Part model, mm, in its own coordinate system. Face numbers are marked on the shaded views. A direction names the side the tool comes from. Round coordinates to 2 decimals unless told otherwise and drop trailing zeros. Write each loop counter-clockwise with the first axis right and the second up, starting at its lowest first coordinate (ties: lowest second). Pieces come first, ordered by that corner, then holes.
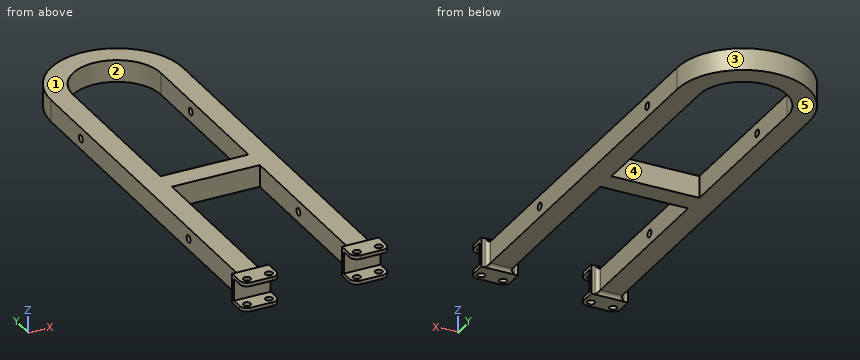
```python
from build123d import *

# Parameters (mm, degrees)
SKETCH1_R               = 5
BOSS_EXTRUDE1_DEPTH     = 50
SKETCH2_W               = 30
SKETCH2_H               = 30
CUT_EXTRUDE1_DEPTH      = 639.479639456
SKETCH3_W               = 30
SKETCH3_H               = 30
SKETCH3_W_2             = 5
SKETCH3_H_2             = 35
CUT_EXTRUDE2_DEPTH      = 642.526499842
FILLET1_R               = 5
SKETCH4_R               = 5
CUT_EXTRUDE3_DEPTH      = 639.10755363
SKETCH5_W               = 30
SKETCH5_H               = 30
BOSS_EXTRUDE2_DEPTH     = 120
SKETCH6_W               = 41.881061045
SKETCH6_H               = 38.598384764
CUT_EXTRUDE4_DEPTH      = 642.156182221
SKETCH7_W               = 50
SKETCH7_H               = 40
BOSS_EXTRUDE3_DEPTH     = 30
SKETCH8_R               = 5
CUT_EXTRUDE5_DEPTH      = 617.973459721
FILLET2_R               = 10
SKETCH9_W               = 30
SKETCH9_H               = 25
CUT_EXTRUDE6_DEPTH      = 642.156182221
CUT_EXTRUDE7_DEPTH      = 639.10755363
CUT_EXTRUDE7_DEPTH_BACK = 639.10755363
SKETCH10_R              = 5


with BuildPart() as part:
    # Sketch1 → Boss-Extrude1 (new body)
    with BuildSketch(Plane.XY):
        with BuildLine():
            Line((90, 17.5), (90, 517.5))
            ThreePointArc((90, 517.5), (0, 607.5), (-90, 517.5))
            Line((-90, 517.5), (-90, 17.5))
            Line((-90, 17.5), (-100, 17.5))
            Line((-100, 17.5), (-100, -7.5))
            ThreePointArc((-100, -7.5), (-97.071067812, -14.571067812), (-90, -17.5))
            Line((-90, -17.5), (-60, -17.5))
            ThreePointArc((-60, -17.5), (-52.928932188, -14.571067812), (-50, -7.5))
            Line((-50, -7.5), (-50, 17.5))
            Line((-50, 17.5), (-60, 17.5))
            Line((-60, 17.5), (-60, 517.5))
            ThreePointArc((-60, 517.5), (0, 577.5), (60, 517.5))
            Line((60, 517.5), (60, 17.5))
            Line((60, 17.5), (50, 17.5))
            Line((50, 17.5), (50, -7.5))
            ThreePointArc((50, -7.5), (52.928932188, -14.571067812), (60, -17.5))
            Line((60, -17.5), (90, -17.5))
            ThreePointArc((90, -17.5), (97.071067812, -14.571067812), (100, -7.5))
            Line((100, -7.5), (100, 17.5))
            Line((100, 17.5), (90, 17.5))
        make_face()
        with Locations((90, -7.5)):
            Circle(SKETCH1_R, mode=Mode.SUBTRACT)
        with Locations((60, -7.5)):
            Circle(SKETCH1_R, mode=Mode.SUBTRACT)
        with Locations((-90, -7.5)):
            Circle(SKETCH1_R, mode=Mode.SUBTRACT)
        with Locations((-60, -7.5)):
            Circle(SKETCH1_R, mode=Mode.SUBTRACT)
    extrude(amount=BOSS_EXTRUDE1_DEPTH)

    # Sketch2 → Cut-Extrude1 (cut, through all)
    with BuildSketch(Plane(origin=(90, 0, 0), x_dir=(0, 0, -1), z_dir=(1, 0, 0))):
        with BuildLine():
            Line((-50, 17.5), (-45, 17.5))
            ThreePointArc((-45, 17.5), (-41.464466094, 18.964466094), (-40, 22.5))
            Line((-40, 22.5), (-40, 607.5))
            Line((-40, 607.5), (-50, 607.5))
            Line((-50, 607.5), (-50, 17.5))
        make_face()
        with Locations((-25, -2.5)):
            Rectangle(SKETCH2_W, SKETCH2_H)
        with BuildLine():
            Line((-5, 17.5), (0, 17.5))
            Line((0, 17.5), (0, 607.5))
            Line((0, 607.5), (-10, 607.5))
            Line((-10, 607.5), (-10, 22.5))
            ThreePointArc((-10, 22.5), (-8.535533906, 18.964466094), (-5, 17.5))
        make_face()
    extrude(amount=-CUT_EXTRUDE1_DEPTH, mode=Mode.SUBTRACT)

    # Sketch3 → Cut-Extrude2 (cut, through all)
    with BuildSketch(Plane(origin=(100, 0, 0), x_dir=(0, 0, -1), z_dir=(1, 0, 0))):
        with Locations((-25, -2.5)):
            Rectangle(SKETCH3_W, SKETCH3_H)
        with Locations((-47.5, 0)):
            Rectangle(SKETCH3_W_2, SKETCH3_H_2)
        with Locations((-2.5, 0)):
            Rectangle(SKETCH3_W_2, SKETCH3_H_2)
    extrude(amount=-CUT_EXTRUDE2_DEPTH, mode=Mode.SUBTRACT)

    # Fillet1
    # the kernel refuses this fillet: 5 mm, written as the material it adds along each edge
    with BuildSketch(Plane(origin=(-90, 17.5, 5), x_dir=(-1, 0, 0), z_dir=(0, 0, 1))) as fillet1_piece_1_section:
        with BuildLine():
            CenterArc((FILLET1_R, -FILLET1_R), FILLET1_R, 90, 90)
            Line((0, -FILLET1_R), (0, 0))
            Line((0, 0), (FILLET1_R, 0))
        make_face()
    fillet1_piece_1 = extrude(amount=40, mode=Mode.PRIVATE)
    fillet1_piece_1 = fillet1_piece_1 - Plane(origin=(-91.427889151, 22.5, 45), x_dir=(0, -1, 0), z_dir=(1, 0, 0)) * Cylinder(5, 101, mode=Mode.PRIVATE)
    fillet1_piece_1 = fillet1_piece_1 - Plane(origin=(-91.427889151, 22.5, 5), x_dir=(0, 0, 1), z_dir=(1, 0, 0)) * Cylinder(5, 101, mode=Mode.PRIVATE)
    add(fillet1_piece_1)
    with BuildSketch(Plane(origin=(60, 17.5, 5), x_dir=(-1, 0, 0), z_dir=(0, 0, 1))) as fillet1_piece_2_section:
        with BuildLine():
            CenterArc((FILLET1_R, -FILLET1_R), FILLET1_R, 90, 90)
            Line((0, -FILLET1_R), (0, 0))
            Line((0, 0), (FILLET1_R, 0))
        make_face()
    fillet1_piece_2 = extrude(amount=40, mode=Mode.PRIVATE)
    fillet1_piece_2 = fillet1_piece_2 - Plane(origin=(58.572110849, 22.5, 5), x_dir=(0, 0, 1), z_dir=(1, 0, 0)) * Cylinder(5, 101, mode=Mode.PRIVATE)
    fillet1_piece_2 = fillet1_piece_2 - Plane(origin=(58.572110849, 22.5, 45), x_dir=(0, -1, 0), z_dir=(1, 0, 0)) * Cylinder(5, 101, mode=Mode.PRIVATE)
    add(fillet1_piece_2)
    with BuildSketch(Plane(origin=(-60, 17.5, 5), x_dir=(1, 0, 0), z_dir=(0, 0, 1))) as fillet1_piece_3_section:
        with BuildLine():
            CenterArc((FILLET1_R, FILLET1_R), FILLET1_R, 180, 90)
            Line((0, FILLET1_R), (0, 0))
            Line((0, 0), (FILLET1_R, 0))
        make_face()
    fillet1_piece_3 = extrude(amount=40, mode=Mode.PRIVATE)
    fillet1_piece_3 = fillet1_piece_3 - Plane(origin=(-58.572110849, 22.5, 45), x_dir=(0, -1, 0), z_dir=(1, 0, 0)) * Cylinder(5, 101, mode=Mode.PRIVATE)
    fillet1_piece_3 = fillet1_piece_3 - Plane(origin=(-58.572110849, 22.5, 5), x_dir=(0, 0, 1), z_dir=(1, 0, 0)) * Cylinder(5, 101, mode=Mode.PRIVATE)
    add(fillet1_piece_3)
    with BuildSketch(Plane(origin=(90, 17.5, 5), x_dir=(0, 1, 0), z_dir=(0, 0, 1))) as fillet1_piece_4_section:
        with BuildLine():
            CenterArc((FILLET1_R, -FILLET1_R), FILLET1_R, 90, 90)
            Line((0, -FILLET1_R), (0, 0))
            Line((0, 0), (FILLET1_R, 0))
        make_face()
    fillet1_piece_4 = extrude(amount=40, mode=Mode.PRIVATE)
    fillet1_piece_4 = fillet1_piece_4 - Plane(origin=(91.427889151, 22.5, 5), x_dir=(0, 0, 1), z_dir=(1, 0, 0)) * Cylinder(5, 101, mode=Mode.PRIVATE)
    fillet1_piece_4 = fillet1_piece_4 - Plane(origin=(91.427889151, 22.5, 45), x_dir=(0, -1, 0), z_dir=(1, 0, 0)) * Cylinder(5, 101, mode=Mode.PRIVATE)
    add(fillet1_piece_4)

    # Sketch4 → Cut-Extrude3 (cut, through all)
    with BuildSketch(Plane(origin=(90, 0, 0), x_dir=(0, 0, -1), z_dir=(1, 0, 0))):
        with Locations(Location((-25, 152.5, 0), (0, 0, 90))):
            Circle(SKETCH4_R)
    extrude(amount=-CUT_EXTRUDE3_DEPTH, mode=Mode.SUBTRACT)

    # Sketch5 → Boss-Extrude2 (add)
    with BuildSketch(Plane(origin=(-60, 0, 0), x_dir=(0, 0, -1), z_dir=(1, 0, 0))):
        with Locations((-25, 270)):
            Rectangle(SKETCH5_W, SKETCH5_H)
    extrude(amount=BOSS_EXTRUDE2_DEPTH)

    # Sketch6 → Cut-Extrude4 (cut, through all)
    with BuildSketch(Plane(origin=(100, 0, 0), x_dir=(0, 0, -1), z_dir=(1, 0, 0))):
        with Locations((-24.059469477, -1.799192382)):
            Rectangle(SKETCH6_W, SKETCH6_H)
    extrude(amount=-CUT_EXTRUDE4_DEPTH, mode=Mode.SUBTRACT)

    # Sketch7 → Boss-Extrude3 (add)
    with BuildSketch(Plane.XZ.offset(-17.5)):
        with Locations((-75, 25)):
            Rectangle(SKETCH7_W, SKETCH7_H)
        with Locations((75, 25)):
            Rectangle(SKETCH7_W, SKETCH7_H)
    extrude(amount=BOSS_EXTRUDE3_DEPTH)

    # Sketch8 → Cut-Extrude5 (cut, through all)
    with BuildSketch(Plane.XY.offset(45)):
        with Locations((-90, -2.5)):
            Circle(SKETCH8_R)
        with Locations((-60, -2.5)):
            Circle(SKETCH8_R)
        with Locations((60, -2.5)):
            Circle(SKETCH8_R)
        with Locations((90, -2.5)):
            Circle(SKETCH8_R)
    extrude(amount=-CUT_EXTRUDE5_DEPTH, mode=Mode.SUBTRACT)

    # Fillet2
    fillet2_edges = [part.edges().sort_by_distance(p)[0] for p in [
        (-100, -12.5, 25),
        (-50, -12.5, 25),
        (50, -12.5, 25),
        (100, -12.5, 25),
    ]]
    fillet(fillet2_edges, radius=FILLET2_R)

    # Sketch9 → Cut-Extrude6 (cut, through all)
    with BuildSketch(Plane.ZY.offset(100)):
        with Locations((25, 0)):
            Rectangle(SKETCH9_W, SKETCH9_H)
    extrude(amount=-CUT_EXTRUDE6_DEPTH, mode=Mode.SUBTRACT)

    # Sketch10 → Cut-Extrude7 (cut, two sides: drawn at the far end of the back side and taken through both)
    with BuildSketch(Plane.ZY.offset(90).offset(-CUT_EXTRUDE7_DEPTH_BACK)):
        with Locations(Location((25, 438.296527551, 0), (0, 0, 270))):
            Circle(SKETCH10_R)
    extrude(amount=CUT_EXTRUDE7_DEPTH + CUT_EXTRUDE7_DEPTH_BACK, mode=Mode.SUBTRACT)


solid = part.part
```
Q1. Cut at B-B on x = 26.5. Write the cut outline in (y, z), plus the area to 3 significant figures.
Values follow:
outline: (255, 10) - (285, 10) - (285, 40) - (255, 40) - close; (571.33, 10) - (603.51, 10) - (603.51, 40) - (571.33, 40) - close
area: 1,870 mm2
Q2. Which spindle directions (+Z, -Z, +X, -X, +Y, -Y) get a long thin tool onto all of the face, cutting with end or side? Do the marked faces 1 and 2. Say none if no direction does.
Values follow:
face 1: +Z, +X, -X, +Y
face 2: +Z, -Z
Q3. Cut at C-C on y = 268. Write the cut outline in (x, z).
Values follow:
outline: (-90, 10) - (90, 10) - (90, 40) - (-90, 40) - close
Q4. Cut at A-A on y = 498. Write the cut outline in (x, z).
Values follow:
outline: (-90, 10) - (-60, 10) - (-60, 40) - (-90, 40) - close; (60, 10) - (90, 10) - (90, 40) - (60, 40) - close
Q5. Wall check: L1, parallel to X at y = -2, z = 8; L2, parallel to X at y = 297, z = 18; L3, parallel to Z at x = -66.25, y = 152.5. Give the ranges that are in metal, low to high.
Values follow:
L1: x = -100 to -94.97, -85.03 to -64.97, -55.03 to -50, 50 to 55.03, 64.97 to 85.03, 94.97 to 100
L2: x = -90 to -60, 60 to 90
L3: z = 10 to 20, 30 to 40
Q6. Mould opens along X. For the marked faces 3, 4 and 5 say: +X half, -X half, draft (parallel to the pull), parting line (faces both ways), or undercut.
Values follow:
face 3: parting line
face 4: undercut
face 5: draft
Q7. Drop flat-ended pins along their axis: pin 1 (8 mm diameter, centred on y = 198, z = 17.5, fed in from +X); pin 2 (2 mm diameter, centred on x = -62.5, z = 29.5, fed in from +Y); pin 3 (15 mm diameter, centred on x = 85, z = 32, fed in from -Y); pin 4 (9 mm diameter, centred on x = -90, y = -2.5, fed in from -Z). Give the stop position or say it passes through.
Values follow:
pin 1: stops at x = 90
pin 2: stops at y = 583.21
pin 3: stops at y = 12.5
pin 4: passes through
